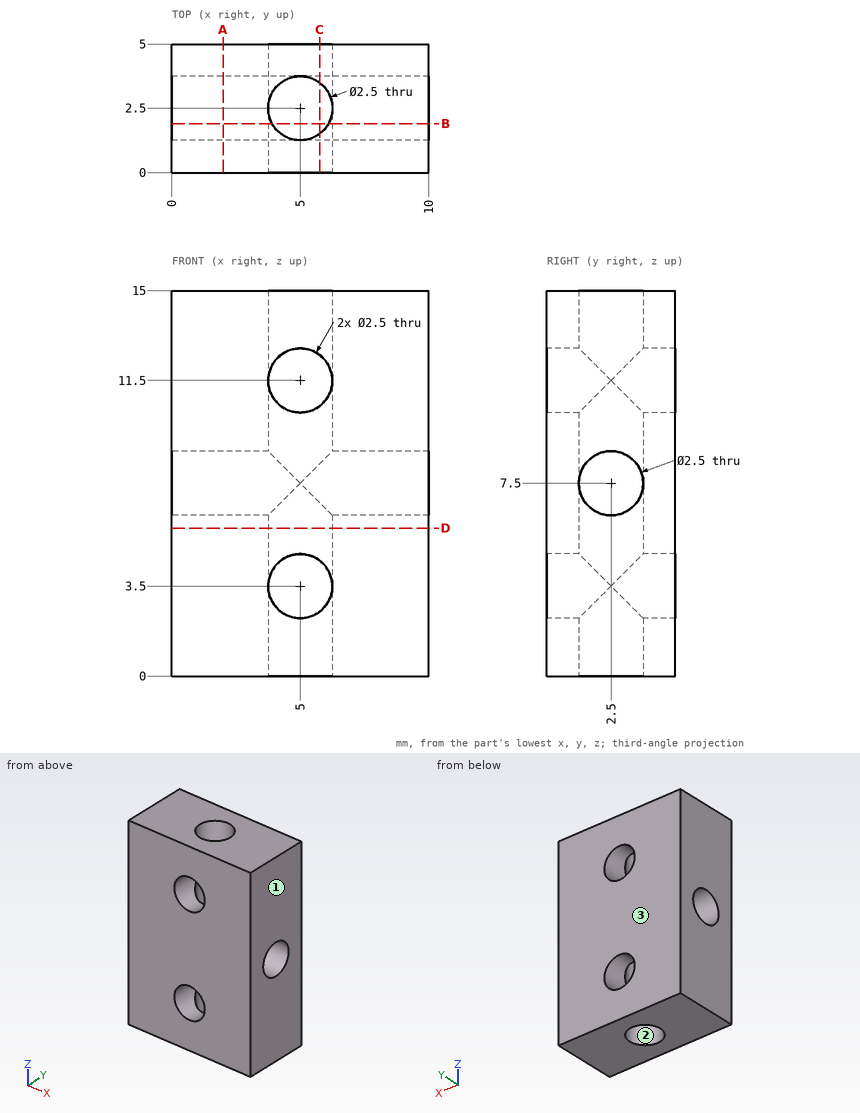
Study the drawing (mm; zero at the part's minimum x, y, z) and answer. Give positions to 0.01 mm unless a question says otherwise; leave off trailing zeros. Write each loop counter-clockwise with the first axis right and the second up, starting at its lowest first coordinate (ties: lowest second). Pieces come first, ordered by that corner, then holes. Notation, with made-up numbers: (78.25, 5) -> (119.25, 5) arc R27 cw to (119.25, 30) -> close; hole circle Ø4 at (70, 66). An arc over 180 degrees is marked (long way). Answer as a JSON object with one key per item and string values. Group by question number.
1) Find section C-C (x = 5.75). Write down the section's boundary in (y, z).
2) Find section D-D (z = 5.75). Write down the section's boundary in (x, y), and give its area (3 significant figures).
3) Find section A-A (x = 2). Write down the section's boundary in (y, z), and give its area (3 significant figures).
4) The mould has two halves that part along Y. Classify the marked faces 1, 2 and 3: +Y half, -Y half, draft (parallel to the pull), parting line (faces both ways), or undercut.
5) Find section B-B (y = 1.9). Write down the section's boundary in (x, z).
6) Consider L1, parallel to Z at x = 5, y = 4.15; L2, parallel to Y at x = 5, z = 9.75; L3, parallel to X at y = 0.8, z = 3.5. Determine where each line is inside the solid, lowest interval first. Write a range as from..to.
7) This flat-tipped pin is pushed along its axis until it touches: P1, Ø1.5, axis at x = 5.5, z = 3, coming from the -Y side. Where does it stop, or does it pass through?
Values follow:
{
 "1": {"outline": "(0, 0) -> (1.5, 0) -> (1.5, 2.5) -> (0, 2.5) -> close; (0, 4.5) -> (1.5, 4.5) -> (1.5, 6.75) arc R1.25 cw to (1.5, 8.25) -> (1.5, 10.5) -> (0, 10.5) -> close; (0, 12.5) -> (1.5, 12.5) -> (1.5, 15) -> (0, 15) -> close; (3.5, 0) -> (5, 0) -> (5, 2.5) -> (3.5, 2.5) -> close; (3.5, 4.5) -> (5, 4.5) -> (5, 10.5) -> (3.5, 10.5) -> (3.5, 8.25) arc R1.25 cw to (3.5, 6.75) -> close; (3.5, 12.5) -> (5, 12.5) -> (5, 15) -> (3.5, 15) -> close"},
 "2": {"outline": "(0, 0) -> (10, 0) -> (10, 5) -> (0, 5) -> close; hole circle Ø2.5 at (5, 2.5)", "area": "45.1 mm2"},
 "3": {"outline": "(0, 0) -> (5, 0) -> (5, 15) -> (0, 15) -> close; hole circle Ø2.5 at (2.5, 7.5)", "area": "70.1 mm2"},
 "4": {"face 1": "draft", "face 2": "undercut", "face 3": "+Y half"},
 "5": {"outline": "(0, 0) -> (3.9, 0) -> (3.9, 2.9) arc R1.25 cw to (3.9, 4.1) -> (3.9, 6.4) -> (0, 6.4) -> close; (0, 8.6) -> (3.9, 8.6) -> (3.9, 10.9) arc R1.25 cw to (3.9, 12.1) -> (3.9, 15) -> (0, 15) -> close; (6.1, 0) -> (10, 0) -> (10, 6.4) -> (6.1, 6.4) -> (6.1, 4.1) arc R1.25 cw to (6.1, 2.9) -> close; (6.1, 8.6) -> (10, 8.6) -> (10, 15) -> (6.1, 15) -> (6.1, 12.1) arc R1.25 cw to (6.1, 10.9) -> close"},
 "6": {"L1": "z = 0..2.25, 4.75..10.25, 12.75..15", "L2": "y = 0..1.25, 3.75..5", "L3": "x = 0..3.75, 6.25..10"},
 "7": {"P1": "stops at y = 0"}
}
